```python
from build123d import *

# Parameters (mm, degrees)
BOSS_EXTRUDE1_DEPTH = 3.35
CUT_EXTRUDE1_REACH  = 5.35
SKETCH2_R           = 2.4


with BuildPart() as part:
    # Sketch1 → Boss-Extrude1 (new body)
    with BuildSketch(Plane(origin=(0, 0, 0), x_dir=(1, 0, 0), z_dir=(0, 1, 0))):
        Polygon((0, 4.907477288), (-4.25, 2.453738644), (-4.25, -2.453738644), (0, -4.907477288), (4.25, -2.453738644), (4.25, 2.453738644), align=None)
    extrude(amount=BOSS_EXTRUDE1_DEPTH)

    # Sketch2 → Cut-Extrude1 (cut, up to next)
    with BuildSketch(Plane(origin=(0, 3.35, 0), x_dir=(1, 0, 0), z_dir=(0, 1, 0)), mode=Mode.PRIVATE) as cut_extrude1_sk1:
        Circle(SKETCH2_R)
    cut_extrude1_tool1 = extrude(cut_extrude1_sk1.sketch, amount=-CUT_EXTRUDE1_REACH, mode=Mode.PRIVATE) & part.part
    add(cut_extrude1_tool1.solids().sort_by_distance((0, 3.35, 0))[0], mode=Mode.SUBTRACT)


solid = part.part
```
Can you work these out from the model? Positions are in its coordinate system, mm. Coordinates: 2 decimals unless noted, no trailing zeros. Loops run counter-clockwise (first coordinate to the right, second up) from the corner with the lowest first, then second, coordinate; pieces in that order, holes last.
1) I need wall thicknesses on probe 1 along X at (y, z) = (2.65, 0); probe 2 along X at (y, z) = (2.3, 1.5); probe 3 along Z at (x, y) = (2, 0.8). Which ranges of each line are inside material? Lowest first, please.
2) Imagine slicing it at C-C on x = 0.75. List the corners of the cut face in (y, z) for me.
3) Imagine slicing it at B-B on z = 0. List the corners of the cut face in (x, y) for me.
4) Thinking about a two-plate mould opening in X: for faces 1 (the flat face through (-2.095, 1.652, -3.698)), 2 (the flat face through (2, 0, 2)), 3 (the flat face through (2.095, 1.652, 3.698)), 4 (the cylindrical face through (1.29, 1.698, -2.024)), which applies, pulls with the +X half, pulls with the -X half, needs draft (parallel to the pull), parting line crosses it, or undercut?
5) Imagine slicing it at D-D on x = 3. List the corners of the cut face in (y, z) for me, plus the area to 3 significant figures.
6) Imagine slicing it at A-A on y = 0.65. List the corners of the cut face in (x, z) for me, plus the area to 3 significant figures.
7) For pin 1 (1 mm diameter, centred on x = -2.5, y = 1, fed in from +Z), with a flat end and sliding along its axis, tell me the tip position at first contact or that it passes through.
Completed:
1. probe 1: x = -4.25 to -2.4, 2.4 to 4.25
1. probe 2: x = -4.25 to -1.87, 1.87 to 4.25
1. probe 3: z = -3.75 to -1.33, 1.33 to 3.75
2. outline: (0, -4.47) - (3.35, -4.47) - (3.35, -2.28) - (0, -2.28) - close; (0, 2.28) - (3.35, 2.28) - (3.35, 4.47) - (0, 4.47) - close
3. outline: (-4.25, 0) - (-2.4, 0) - (-2.4, 3.35) - (-4.25, 3.35) - close; (2.4, 0) - (4.25, 0) - (4.25, 3.35) - (2.4, 3.35) - close
4. face 1: pulls with the -X half
4. face 2: needs draft
4. face 3: pulls with the +X half
4. face 4: undercut
5. outline: (0, -3.18) - (3.35, -3.18) - (3.35, 3.18) - (0, 3.18) - close
5. area: 21.3 mm2
6. outline: (-4.25, -2.45) - (0, -4.91) - (4.25, -2.45) - (4.25, 2.45) - (0, 4.91) - (-4.25, 2.45) - close; hole circle Ø4.8 at (0, 0)
6. area: 44.5 mm2
7. pin 1: stops at z = 3.75
